CAD build for the part. Positions are in the model's coordinates, mm. Round coordinates to 2 decimals unless told otherwise and drop trailing zeros. Order: outer loops, then holes, each group sorted by start corner. A loop starts at its lowest first (then second) coordinate and runs counter-clockwise, first axis right, second up. Notation, with made-up numbers: M 36.5,12.5 L 58.5,12.5 A34 ccw 58.5,42.5 Z; hole C -18,32 d11. An arc over 180 degrees is marked long. Answer as a JSON object with one key per item and string values.
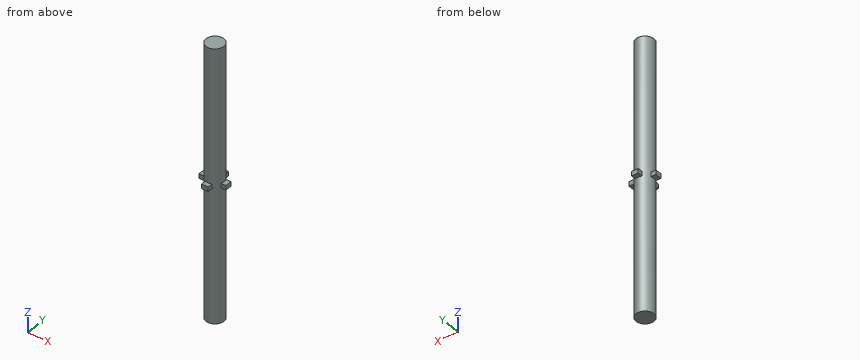
```python
from build123d import *

# Parameters (mm, degrees)
F0_R     = 2.54
F1_DEPTH = 76.2
F4_DEPTH = 0.635


with BuildPart() as f1:
    # F0 (on Top) → F1 (new body)
    with BuildSketch(Plane.XY):
        Circle(F0_R)
    extrude(amount=F1_DEPTH)

    # F3 (on offset) → F4 (join, symmetric)
    with BuildSketch(Plane.XY.offset(38.1)):
        Polygon((0.9525, 0.9525), (0.9525, 3.81), (-0.9525, 3.81), (-0.9525, 0.9525), (-3.81, 0.9525), (-3.81, -0.9525), (-0.9525, -0.9525), (-0.9525, -3.81), (0.9525, -3.81), (0.9525, -0.9525), (3.81, -0.9525), (3.81, 0.9525), align=None)
    extrude(amount=F4_DEPTH, both=True)


solid = f1.part
```
Item 1: Wall check: line 1 along X through (y, z) = (-0.25, 26.5); line 2 along X through (y, z) = (1.75, 58); line 3 along Z through (x, y) = (0.75, 3.5) (3 decimals). Give the ranges that are in metal, low to high. Write a range as [from, to].
Worked answers:
{"line 1": "x = [-2.53, 2.53]", "line 2": "x = [-1.84, 1.84]", "line 3": "z = [37.465, 38.735]"}
Item 2: Saw through at A-A on x = 0. List the corners of the cut face in (y, z) (3 decimals).
Worked answers:
{"outline": "M -3.81,37.465 L -2.54,37.465 L -2.54,0 L 2.54,0 L 2.54,37.465 L 3.81,37.465 L 3.81,38.735 L 2.54,38.735 L 2.54,76.2 L -2.54,76.2 L -2.54,38.735 L -3.81,38.735 Z"}
Item 3: Saw through at C-C on z = 36. List the corners of the cut face in (x, y), and give its area (3 significant figures).
Worked answers:
{"outline": "C 0,0 d5.08", "area": "20.3 mm2"}
Item 4: Drop flat-ended pins along their axis: pin 1 Ø4 at (x, z) = (-1.5, 55) entering from -Y; pin 2 Ø0.7 at (x, y) = (-3, -0.5) entering from +Z (3 decimals); pin 3 Ø1 at (y, z) = (3, 38) entering from +X. Give the stop position or say it passes through.
Worked answers:
{"pin 1": "stops at y = -2.54", "pin 2": "stops at z = 38.735", "pin 3": "stops at x = 0.95"}
